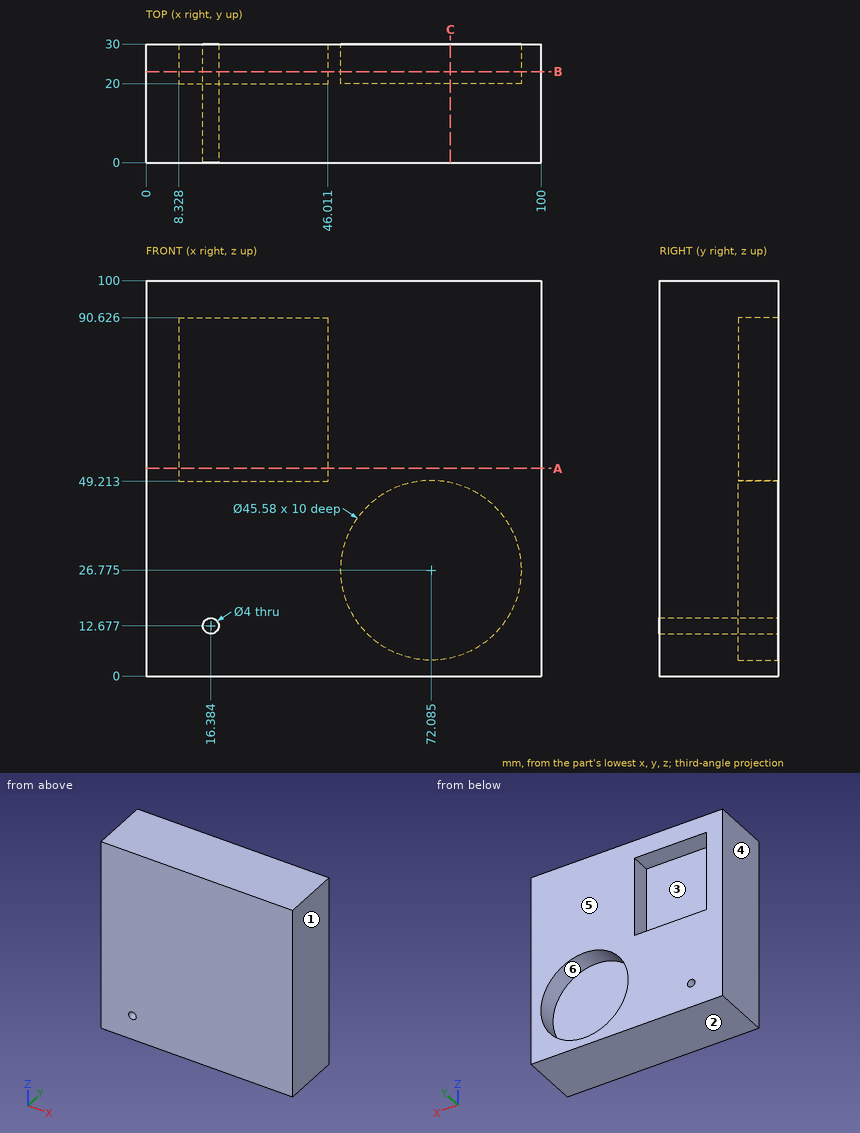
Drawing for the job (mm, zero at the part's lowest x, y, z). A direction names the side the tool comes from. Round coordinates to 2 decimals unless told otherwise and drop trailing zeros. Loops run counter-clockwise (first coordinate to the right, second up) from the corner with the lowest first, then second, coordinate; pieces in that order, holes last. Notation, with made-up numbers: (23.25, 9.25) -> (49.25, 9.25) arc R22 cw to (49.25, 31.25) -> close; hole circle Ø4 at (-34.75, 40). An arc over 180 degrees is marked (long way). Answer in a Markdown table with one row per item.
Item 1: Which spindle directions (+Z, -Z, +X, -X, +Y, -Y) get a long thin tool onto all of the face, cutting with end or side? Do the marked faces 5 and 6. Say none if no direction does.
Answers below:
| item | result |
|---|---|
| face 5 | +Z, -Z, +X, -X, +Y |
| face 6 | +Y |
Item 2: Saw through at A-A (z = 52.5). Write the cut outline in (x, y).
Answers below:
| item | result |
|---|---|
| outline | (0, 0) -> (100, 0) -> (100, 30) -> (46.01, 30) -> (46.01, 20) -> (8.33, 20) -> (8.33, 30) -> (0, 30) -> close |
Item 3: Pin check, flat tip, straight feed: pin 1 (12 mm diameter, centred on x = 64, z = 58, fed in from -Y). Stop position of the tip, or through.
Answers below:
| item | result |
|---|---|
| pin 1 | stops at y = 0 |
Item 4: Mould opens along X. For the marked faces 1, 2, 3 and 4 say: +X half, -X half, draft (parallel to the pull), parting line (faces both ways), or undercut.
Answers below:
| item | result |
|---|---|
| face 1 | +X half |
| face 2 | draft |
| face 3 | undercut |
| face 4 | -X half |
Item 5: Saw through at C-C (x = 77). Write the cut outline in (y, z), and give its area (4 significant figures).
Answers below:
| item | result |
|---|---|
| outline | (0, 0) -> (30, 0) -> (30, 4.52) -> (20, 4.52) -> (20, 49.03) -> (30, 49.03) -> (30, 100) -> (0, 100) -> close |
| area | 2,555 mm² |
Item 6: Saw through at B-B (y = 23). Write the cut outline in (x, z) (1 decimal).
Answers below:
| item | result |
|---|---|
| outline | (0, 0) -> (100, 0) -> (100, 100) -> (0, 100) -> close; hole (8.3, 49.2) -> (46, 49.2) -> (46, 90.6) -> (8.3, 90.6) -> close; hole circle Ø4 at (16.4, 12.7); hole circle Ø45.6 at (72.1, 26.8) |
Item 7: Drill centre lines: L1, parallel to X at y = 27.75, z = 85; L2, parallel to Z at x = 16.5, y = 2.5; L3, parallel to Z at x = 26, y = 21.25. Where is each one in solid material? Low to high. Write a range as [from, to].
Answers below:
| item | result |
|---|---|
| L1 | x = [0, 8.33], [46.01, 100] |
| L2 | z = [0, 10.68], [14.67, 100] |
| L3 | z = [0, 49.21], [90.63, 100] |
